For this review, take the finished solid that the model builds, in its own axes (mm). Face numbers are marked on the shaded views. A direction names the side the tool comes from. Give positions to 0.01 mm unless a question says otherwise; leave off trailing zeros. Loops run counter-clockwise (first coordinate to the right, second up) from the corner with the lowest first, then second, coordinate; pieces in that order, holes last. Notation, with made-up numbers: (12.5, 2) - (68.5, 2) arc R26 cw to (68.5, 34) - close; hole circle Ø9 at (1.5, -15). An arc over 180 degrees is marked (long way). Put each result on its own line as item: value. Start each with the question number.
Solid Edge part; units mm, degrees
sketch "Sketch1" plane through (0, 0, 0) normal (0, -1, 0) x (1, 0, 0)
  line L0 (-12.5, -17.5) -> (12.5, -17.5)
  line L1 (12.5, -17.5) -> (12.5, 17.5)
  line L2 (12.5, 17.5) -> (-12.5, 17.5)
  line L3 (-12.5, 17.5) -> (-12.5, -17.5)
extrude "Protrusion1" add sketch "Sketch1" along normal mid plane 1.5
sketch "Sketch2" plane through (0, -0.75, 0) normal (0, -1, 0) x (1, 0, 0)
  line L0 (8.3607, -9.3028) -> (-8.3607, -9.3028)
  line L1 (-8.3607, -9.3028) -> (-8.3607, 9.3028)
  line L2 (-8.3607, 9.3028) -> (8.3607, 9.3028)
  line L3 (8.3607, 9.3028) -> (8.3607, -9.3028)
extrude "ExtrudedProtrusion_3" add sketch "Sketch2" along normal blind 5 and the other way blind 0.6492
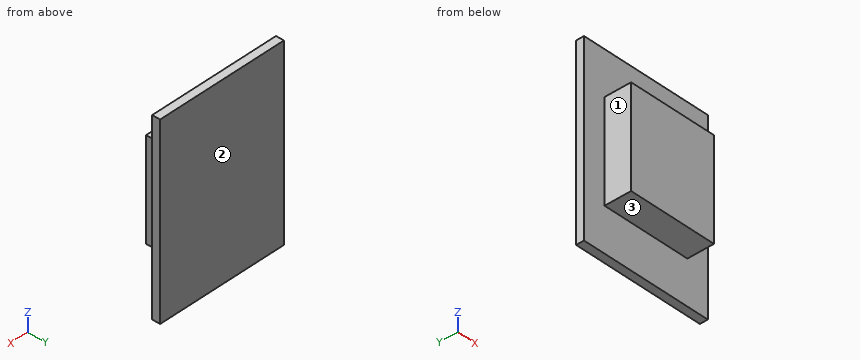
1) Take a section at B-B on x = 3.5. State the section outline as (y, z) points.
2) Wall thickness on probe 1 along Z at (x, y) = (-0.5, -4.25); probe 2 along Y at (x, z) = (10, -9); probe 3 along X at (y, z) = (-4, -4): over which ranges is each line inside the solid? List them lowest first.
3) Machinability: for the marked faces 1, 2 and 3, which of the approach directions +Z, -Z, +X, -X, +Y, -Y give a long, thin tool a straight path to every point of the face, cutting with its end or side? Answer none if there is none.
4) Insertion check: P1, Ø3, axis at x = 3.5, y = -1, coming from the -Z side; P2, Ø1.5, axis at x = 0.5, y = -2.5, coming from the +Z side; P3, Ø1.5, axis at y = -3, z = -4, coming from the +X side; P4, Ø1.5, axis at x = 3, y = -4, coming from the -Z side. Each pin has a flat end and moves straight along its axis. Give the tip position at first contact, or say it passes through.
5) Take a section at A-A on z = -5.5. State the section outline as (x, y) points, and give its area (3 significant figures).
6) Take a section at D-D on z = 11. State the section outline as (x, y) points.
7) Take a section at C-C on y = -4. State the section outline as (x, z) points.
Answers follow:
1. outline: (-5.75, -9.3) - (-0.75, -9.3) - (-0.75, -17.5) - (0.75, -17.5) - (0.75, 17.5) - (-0.75, 17.5) - (-0.75, 9.3) - (-5.75, 9.3) - close
2. probe 1: -9.3 to 9.3
2. probe 2: -0.75 to 0.75
2. probe 3: -8.36 to 8.36
3. face 1: +Z, -Z, -X, -Y
3. face 2: +Z, -Z, +X, -X, +Y
3. face 3: -Z, +X, -X, -Y
4. P1: z = -17.5
4. P2: z = 9.3
4. P3: x = 8.36
4. P4: z = -9.3
5. outline: (-12.5, -0.75) - (-8.36, -0.75) - (-8.36, -5.75) - (8.36, -5.75) - (8.36, -0.75) - (12.5, -0.75) - (12.5, 0.75) - (-12.5, 0.75) - close
5. area: 121 mm2
6. outline: (-12.5, -0.75) - (12.5, -0.75) - (12.5, 0.75) - (-12.5, 0.75) - close
7. outline: (-8.36, -9.3) - (8.36, -9.3) - (8.36, 9.3) - (-8.36, 9.3) - close
